from build123d import *

# Parameters (mm, degrees)
ESQUISSE1_R             = 30.1
ESQUISSE1_R_2           = 2.25
ESQUISSE1_R_3           = 8.1
BOSS_EXTRU_1_DEPTH      = 10
ESQUISSE2_R             = 8.1
ESQUISSE2_R_2           = 5.5
BOSS_EXTRU_2_DEPTH      = 4.5
ESQUISSE3_R             = 4.5
ENL_V_MAT_EXTRU_1_DEPTH = 3.5
ESQUISSE4_R             = 42.1
ESQUISSE4_R_2           = 30.1
BOSS_EXTRU_3_DEPTH      = 6
BOSS_EXTRU_4_START      = 9
ESQUISSE6_R             = 37.5
ESQUISSE6_R_2           = 30.1
BOSS_EXTRU_4_DEPTH      = 9


with BuildPart() as part:
    # Esquisse1 → Boss.-Extru.1 (new body)
    with BuildSketch(Plane.XY):
        Circle(ESQUISSE1_R)
        with Locations((22, 0)):
            Circle(ESQUISSE1_R_2, mode=Mode.SUBTRACT)
        with Locations((11, -19.052558883)):
            Circle(ESQUISSE1_R_2, mode=Mode.SUBTRACT)
        with Locations((-11, -19.052558883)):
            Circle(ESQUISSE1_R_2, mode=Mode.SUBTRACT)
        with Locations((-22, 0)):
            Circle(ESQUISSE1_R_2, mode=Mode.SUBTRACT)
        with Locations((-11, 19.052558883)):
            Circle(ESQUISSE1_R_2, mode=Mode.SUBTRACT)
        with Locations((11, 19.052558883)):
            Circle(ESQUISSE1_R_2, mode=Mode.SUBTRACT)
        Circle(ESQUISSE1_R_3, mode=Mode.SUBTRACT)
    extrude(amount=BOSS_EXTRU_1_DEPTH)

    # Esquisse2 → Boss.-Extru.2 (add)
    with BuildSketch(Plane(origin=(0, 0, 0), x_dir=(-1, 0, 0), z_dir=(0, 0, -1))):
        Circle(ESQUISSE2_R)
        Circle(ESQUISSE2_R_2, mode=Mode.SUBTRACT)
    extrude(amount=-BOSS_EXTRU_2_DEPTH)

    # Esquisse3 → Enlèv. mat.-Extru.1 (cut)
    with BuildSketch(Plane.XY.offset(10)):
        with Locations((-11, 19.052558883)):
            Circle(ESQUISSE3_R)
        with Locations((11, 19.052558883)):
            Circle(ESQUISSE3_R)
        with Locations((22, 0)):
            Circle(ESQUISSE3_R)
        with Locations((11, -19.052558883)):
            Circle(ESQUISSE3_R)
        with Locations((-11, -19.052558883)):
            Circle(ESQUISSE3_R)
        with Locations((-22, 0)):
            Circle(ESQUISSE3_R)
    extrude(amount=-ENL_V_MAT_EXTRU_1_DEPTH, mode=Mode.SUBTRACT)



with BuildPart() as body_2:
    # Esquisse4 → Boss.-Extru.3 (new body)
    with BuildSketch(Plane.XY.offset(10)):
        Circle(ESQUISSE4_R)
        Circle(ESQUISSE4_R_2, mode=Mode.SUBTRACT)
    extrude(amount=BOSS_EXTRU_3_DEPTH)


with BuildPart() as part_1:
    add(part.part)

    add(body_2.part)  # Boss.-Extru.4 merges body 2
    # Esquisse6 → Boss.-Extru.4 (add)
    with BuildSketch(Plane(origin=(0, 0, 10), x_dir=(-1, 0, 0), z_dir=(0, 0, -1)).offset(BOSS_EXTRU_4_START)):
        Circle(ESQUISSE6_R)
        Circle(ESQUISSE6_R_2, mode=Mode.SUBTRACT)
    extrude(amount=-BOSS_EXTRU_4_DEPTH)


solid = part_1.part
The listing builds one solid part. Answer for the finished solid, in the listing's coordinates (mm). A direction names the side the tool comes from. Coordinates: 2 decimals unless noted, no trailing zeros. Loops run counter-clockwise (first coordinate to the right, second up) from the corner with the lowest first, then second, coordinate; pieces in that order, holes last. Notation, with made-up numbers: (66, 58.5) -> (76, 58.5) arc R30 ccw to (76, 86.5) -> close; hole circle Ø8 at (-2.5, -21.5). An arc over 180 degrees is marked (long way). Answer in a Markdown table with one row per item. Add a question column.
1. For faces 1 (the cylindrical face through (10.71, -16.82, 3.2)), 2 (the cylindrical face through (4.88, 37.18, 5.44)), 3 (the cylindrical face through (-26.496, 0.198, 8.274)), determine the directions among +Z, -Z, +X, -X, +Y, -Y from which every point of the face is accessible in a straight line to the end or side of a thin tool.
2. Consider line 1 (X direction, y = -23, z = 8); line 2 (X direction, y = 1, z = 1.5); line 3 (Z direction, x = 13, y = 12). Determine where each line is inside the solid, lowest interval first. Write a range as [from, to].
3. Determine the mould class of faces 4 (the flat face through (-6, 0, 0)), 5 (the cylindrical face through (-6.525, -29.384, 0.493)), 6 (the cylindrical face through (-11.29, -16.82, 3.2)) for opening direction X: +X half, -X half, draft (parallel to the pull), parting line (faces both ways), or undercut.
4. The part is cut by section A-A, the plane x = 0. Write down the section's boundary in (y, z).
5. The part is cut by section B-B, the plane z = 8.25. Write down the section's boundary in (x, y), then the cut area to 3 significant figures.
6. Flat-ended cylindrical pins translate along their axes: P1, Ø5, axis at x = 11, y = -19.05, coming from the +Z side; P2, Ø1, axis at x = -16, y = -22, coming from the +Z side; P3, Ø6, axis at x = 0, z = 3, coming from the +Y side. Find the tip coordinate at first contact, or state that the pin passes through.
7. The part is cut by section C-C, the plane x = -11. Count the separate pieces of the cut face and the enclosed holes in it, then the cut area to 3 significant figures.
Answer below:
| question | item | result |
|---|---|---|
| 1 | face 1 | +Z, -Z |
| 1 | face 2 | -Z |
| 1 | face 3 | +Z |
| 2 | line 1 | [-29.62, -13.16], [-8.84, 8.84], [13.16, 29.62] |
| 2 | line 2 | [-37.49, -24.02], [-19.98, -5.41], [5.41, 19.98], [24.02, 37.49] |
| 2 | line 3 | [0, 10] |
| 3 | face 4 | draft |
| 3 | face 5 | parting line |
| 3 | face 6 | undercut |
| 4 | outline | (-42.1, 10) -> (-37.5, 10) -> (-37.5, 1) -> (-30.1, 1) -> (-30.1, 0) -> (-5.5, 0) -> (-5.5, 4.5) -> (-8.1, 4.5) -> (-8.1, 10) -> (-30.1, 10) -> (-30.1, 16) -> (-42.1, 16) -> close; (5.5, 0) -> (30.1, 0) -> (30.1, 1) -> (37.5, 1) -> (37.5, 10) -> (42.1, 10) -> (42.1, 16) -> (30.1, 16) -> (30.1, 10) -> (8.1, 10) -> (8.1, 4.5) -> (5.5, 4.5) -> close |
| 5 | outline | circle Ø75 at (0, 0); hole circle Ø9 at (-22, 0); hole circle Ø9 at (-11, -19.05); hole circle Ø9 at (-11, 19.05); hole circle Ø16.2 at (0, 0); hole circle Ø9 at (11, -19.05); hole circle Ø9 at (11, 19.05); hole circle Ø9 at (22, 0) |
| 5 | area | 3,830 mm2 |
| 6 | P1 | z = 6.5 |
| 6 | P2 | z = 10 |
| 6 | P3 | y = 37.5 |
| 7 | separate pieces | 3 |
| 7 | enclosed holes | 0 |
| 7 | area | 731 mm2 |
